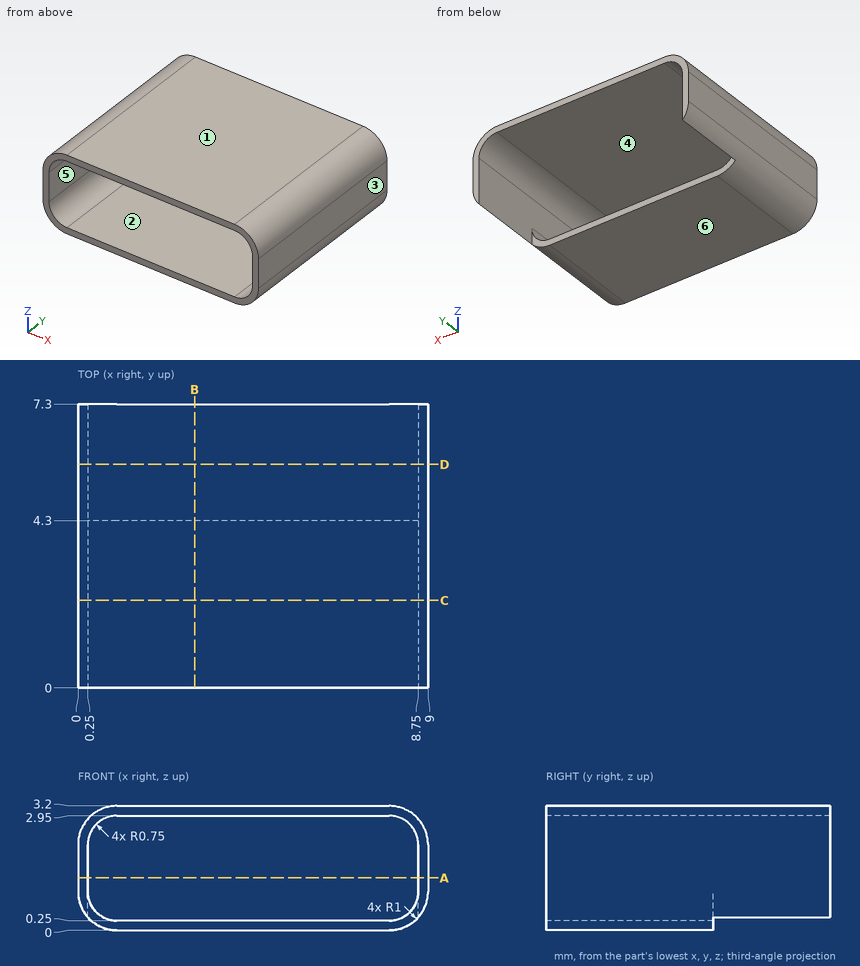
Study the drawing (mm; zero at the part's minimum x, y, z) and answer. A direction names the side the tool comes from. Round coordinates to 2 decimals unless told otherwise and drop trailing zeros. Order: outer loops, then holes, each group sorted by start corner. A loop starts at its lowest first (then second) coordinate and runs counter-clockwise, first axis right, second up. Notation, with made-up numbers: M -21.5,-32 L -1.5,-32 A19 ccw -1.5,-7 Z; hole C -35,88.25 d4. An arc over 180 degrees is marked long. One line per item, written item: value.
Q1. Find section C-C on y = 2.25. Write down the section's boundary in (x, z), then the cut area to 3 significant figures.
Derived:
outline: M 0,1 A1 ccw 1,0 L 8,0 A1 ccw 9,1 L 9,2.2 A1 ccw 8,3.2 L 1,3.2 A1 ccw 0,2.2 Z; hole M 0.25,1 A0.75 ccw 1,0.25 L 8,0.25 A0.75 ccw 8.75,1 L 8.75,2.2 A0.75 ccw 8,2.95 L 1,2.95 A0.75 ccw 0.25,2.2 Z
area: 5.47 mm²
Q2. Find section A-A on z = 1.35. Write down the section's boundary in (x, y), then the cut area to 3 significant figures.
Derived:
outline: M 0,0 L 0.25,0 L 0.25,7.3 L 0,7.3 Z; M 8.75,0 L 9,0 L 9,7.3 L 8.75,7.3 Z
area: 3.65 mm²
Q3. Find section D-D on y = 5.75. Write down the section's boundary in (x, z).
Derived:
outline: M 0,1 A1 ccw 0.25,0.34 L 0.25,2.2 A0.75 cw 1,2.95 L 8,2.95 A0.75 cw 8.75,2.2 L 8.75,0.34 A1 ccw 9,1 L 9,2.2 A1 ccw 8,3.2 L 1,3.2 A1 ccw 0,2.2 Z
Q4. For the marked faces 5 and 6, determine the directions among +Z, -Z, +X, -X, +Y, -Y from which every point of the face is accessible in a straight line to the end or side of a thin tool.
Derived:
face 5: +Y
face 6: -Z, +X, -X, +Y, -Y
Q5. Determine the mould class of the marked faces 1, 2, 3 and 4 for opening direction Z: released by +Z, released by -Z, zero draft, split by the parting line, or undercut.
Derived:
face 1: released by +Z
face 2: undercut
face 3: zero draft
face 4: undercut
Q6. Find section B-B on x = 3. Write down the section's boundary in (y, z).
Derived:
outline: M 0,0 L 4.3,0 L 4.3,0.25 L 0,0.25 Z; M 0,2.95 L 7.3,2.95 L 7.3,3.2 L 0,3.2 Z
Q7. Straight lines are drawn through the part: line 1 (Z direction, x = 6.5, y = 0.5); line 2 (X direction, y = 6, z = 1.1). For each, find the intervals that lie inside material, in ascending order.
Derived:
line 1: 0 to 0.25, 2.95 to 3.2
line 2: 0 to 0.25, 8.75 to 9
